from build123d import *

# Parameters (mm, degrees)
SKETCH_1_R      = 1.6
EXTRUDE_1_DEPTH = 2


with BuildPart() as part:
    # 草图1 → 凸台-拉伸1 (new body)
    with BuildSketch(Plane(origin=(0, 0, 0), x_dir=(1, 0, 0), z_dir=(0, 1, 0))):
        Polygon((-30, 28.86862915), (-30, 0.8), (-21.23, 0.8), (-21.23, -0.8), (-30, -0.8), (-30, -28.86862915), (-19.758831067, -18.627460217), (-18.627460217, -19.758831067), (-28.86862915, -30), (-0.8, -30), (-0.8, -21.23), (0.8, -21.23), (0.8, -30), (28.86862915, -30), (18.627460217, -19.758831067), (19.758831067, -18.627460217), (30, -28.86862915), (30, -0.8), (21.23, -0.8), (21.23, 0.8), (30, 0.8), (30, 28.86862915), (19.758831067, 18.627460217), (18.627460217, 19.758831067), (28.86862915, 30), (0.8, 30), (0.8, 21.23), (-0.8, 21.23), (-0.8, 30), (-28.86862915, 30), (-18.627460217, 19.758831067), (-19.758831067, 18.627460217), align=None)
        with Locations(Location((0, -8.08, 0), (0, 0, 270))):
            Circle(SKETCH_1_R, mode=Mode.SUBTRACT)
        with Locations(Location((-8.08, 0, 0), (0, 0, 270))):
            Circle(SKETCH_1_R, mode=Mode.SUBTRACT)
        with Locations(Location((8.08, 0, 0), (0, 0, 270))):
            Circle(SKETCH_1_R, mode=Mode.SUBTRACT)
        with Locations(Location((0, 8.08, 0), (0, 0, 270))):
            Circle(SKETCH_1_R, mode=Mode.SUBTRACT)
    extrude(amount=EXTRUDE_1_DEPTH)


solid = part.part
Check sheet for the modelled part. Datum: model origin and axes. Units: mm. A direction names the side the tool comes from. Round coordinates to 2 decimals unless told otherwise and drop trailing zeros. Loops run counter-clockwise (first coordinate to the right, second up) from the corner with the lowest first, then second, coordinate; pieces in that order, holes last. Notation, with made-up numbers: M -3.75,-13.5 L 51.25,-13.5 A16 cw 51.25,-2.5 Z; hole C 20,72.5 d11. An arc over 180 degrees is marked long. One line per item, written item: value.
(1) Thickness scan on line 1 (X direction, y = 0.7, z = 0); line 2 (X direction, y = 0.95, z = 25); line 3 (Z direction, x = 23.5, y = 0.75). Record the ranges inside material, lowest first.
Computed values:
line 1: x = -21.23 to -9.68, -6.48 to 6.48, 9.68 to 21.23
line 2: x = -30 to -26.13, -23.87 to -0.8, 0.8 to 23.87, 26.13 to 30
line 3: z = -30 to -24.63, -22.37 to -0.8, 0.8 to 22.37, 24.63 to 30
(2) Depth check by flat-ended pin: pin 1 Ø0.8 at (x, y) = (0, 1) entering from +Z; pin 2 Ø0.5 at (x, y) = (0, 1) entering from -Z; pin 3 Ø0.5 at (y, z) = (1, 0.5) entering from -X. Enter the tip coordinate at first touch or a pass-through.
Computed values:
pin 1: stops at z = 21.23
pin 2: stops at z = -21.23
pin 3: stops at x = -21.23
(3) Access from +Z, -Z, +X, -X, +Y, -Y to the whole of each face (thin tool, end or side, straight path). Record for faces 1 (the face through (-26, 1, -0.8)), 2 (the face through (0, 0, 0)), 3 (the face through (0.8, 1, 26)), 4 (the face through (-24.81, 0.99, -23.68)), 5 (the face through (0, 1, -21.23)).
Computed values:
face 1: -X, +Y, -Y
face 2: +Z, -Z, +X, -X, -Y
face 3: +Z, +Y, -Y
face 4: +Y, -Y
face 5: -Z, +Y, -Y
(4) Sectioned sample at B-B, the plane x = 0. Record the cut outline in (y, z).
Computed values:
outline: M 0,-21.23 L 2,-21.23 L 2,-9.68 L 0,-9.68 Z; M 0,-6.48 L 2,-6.48 L 2,6.48 L 0,6.48 Z; M 0,9.68 L 2,9.68 L 2,21.23 L 0,21.23 Z
(5) Sectioned sample at D-D, the plane x = 8.08. Record the cut outline in (y, z).
Computed values:
outline: M 0,-30 L 2,-30 L 2,-1.6 L 0,-1.6 Z; M 0,1.6 L 2,1.6 L 2,30 L 0,30 Z
(6) Sectioned sample at C-C, the plane z = 8.08. Record the cut outline in (x, y).
Computed values:
outline: M -30,0 L -1.6,0 L -1.6,2 L -30,2 Z; M 1.6,0 L 30,0 L 30,2 L 1.6,2 Z
(7) Release check for a two-part mould opening along Z. For faces 6 (the face through (23.68, 0.99, -24.81)), 7 (the face through (-0.8, 1, 26)), 8 (the face through (15, 1, -30)), 9 (the face through (0, 1, 21.23)) record: +Z half, -Z half, draft (parallel to the pull), parting line (faces both ways), or undercut.
Computed values:
face 6: undercut
face 7: draft
face 8: -Z half
face 9: +Z half
(8) Sectioned sample at A-A, the plane z = 0. Record the cut outline in (x, y).
Computed values:
outline: M -21.23,0 L -9.68,0 L -9.68,2 L -21.23,2 Z; M -6.48,0 L 6.48,0 L 6.48,2 L -6.48,2 Z; M 9.68,0 L 21.23,0 L 21.23,2 L 9.68,2 Z
